The figure shows three views and two pictorial views of one solid part (mm, origin at its lowest corner). Answer the questions. A direction names the side the tool comes from. Give positions to 0.01 mm unless a question says otherwise; leave off trailing zeros. Loops run counter-clockwise (first coordinate to the right, second up) from the corner with the lowest first, then second, coordinate; pieces in that order, holes last. Notation, with made-up numbers: (75.5, -28.75) -> (113.5, -28.75) arc R21 cw to (113.5, -24.75) -> close; hole circle Ø9 at (72, 39.25). An arc over 180 degrees is marked (long way). Answer as CSV lines item,"result". Start each with the question number.
1. Flat-ended cylindrical pins translate along their axes: pin 1 Ø2.5 at (x, z) = (10, 10) entering from +Y; pin 2 Ø6 at (x, y) = (14.5, 2.5) entering from +Z; pin 3 Ø6 at (x, y) = (10.5, 1.5) entering from -Z; pin 4 Ø2 at (x, z) = (16.5, 3) entering from -Y. Find the tip coordinate at first contact, or state that the pin passes through.
2. Determine the mould class of the marked faces 3, 4, 5 and 6 for opening direction X: +X half, -X half, draft (parallel to the pull), parting line (faces both ways), or undercut.
3. Find section A-A, the plane z = 10. Give the vertices of the cut face in (x, y).
4. Find section D-D, the plane z = 12. Give the vertices of the cut face in (x, y).
5. A tool of negligible diameter and unlimited length cuts with its end or side. For the marked faces 1 and 2, from which of +Z, -Z, +X, -X, +Y, -Y can it reach the whole face along a straight path? Write none if from no direction.
6. Find the intervals of material crossed by line 1 along Y through (x, z) = (12, 4.5); line 2 along X through (y, z) = (2.25, 8.75) (1 decimal); line 3 along X through (y, z) = (9.25, 13), in increasing order.
7. Find section C-C, the plane y = 2. Give the vertices of the cut face in (x, z) (1 decimal).
8. Find section B-B, the plane x = 10. Give the vertices of the cut face in (y, z).
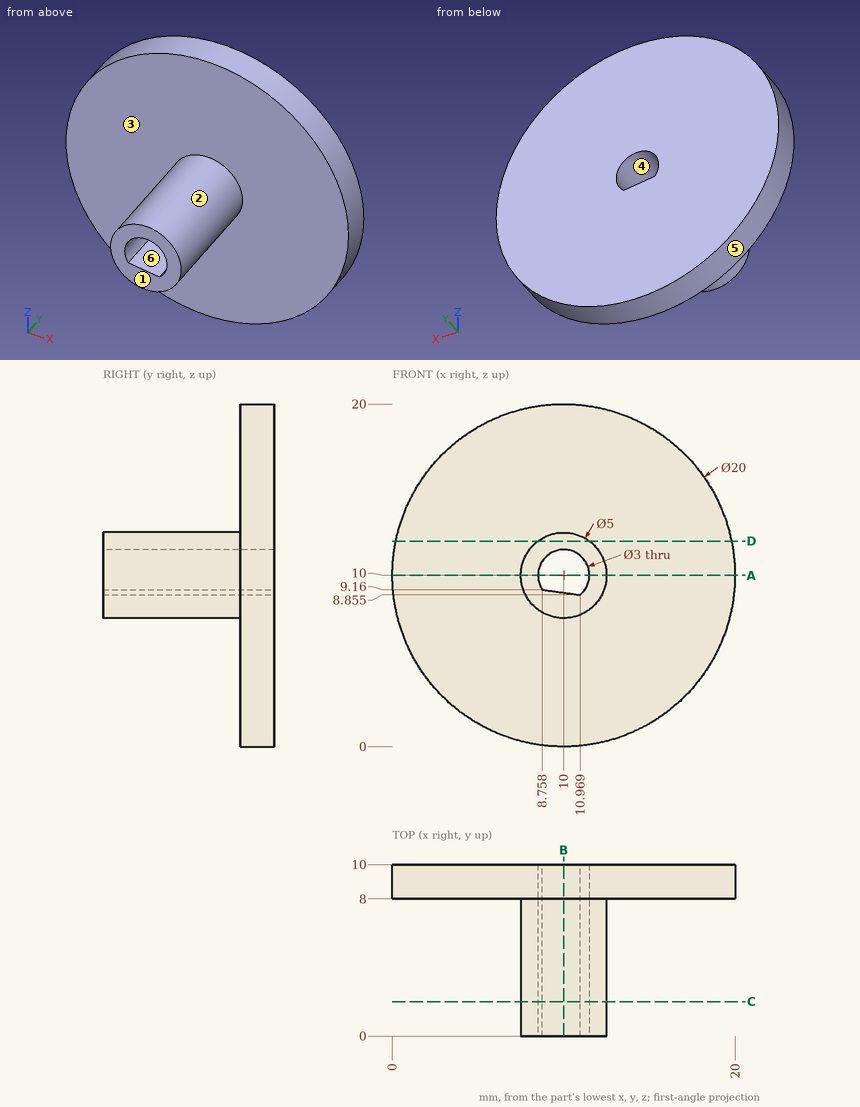
Resolved:
1,pin 1,"stops at y = 10"
1,pin 2,"stops at z = 12"
1,pin 3,"stops at z = 7.5"
1,pin 4,"stops at y = 8"
2,face 3,"draft"
2,face 4,"undercut"
2,face 5,"parting line"
2,face 6,"undercut"
3,outline,"(0, 8) -> (7.5, 8) -> (7.5, 0) -> (8.5, 0) -> (8.5, 10) -> (0, 10) -> close; (11.5, 0) -> (12.5, 0) -> (12.5, 8) -> (20, 8) -> (20, 10) -> (11.5, 10) -> close"
4,outline,"(0.2, 8) -> (8.5, 8) -> (8.5, 0) -> (11.5, 0) -> (11.5, 8) -> (19.8, 8) -> (19.8, 10) -> (0.2, 10) -> close"
5,face 1,"+Z, -Z, +X, -X, -Y"
5,face 2,"-Y"
6,line 1,"y = 8 to 10"
6,line 2,"x = 7.8 to 12.2"
6,line 3,"x = 0.46 to 19.54"
7,outline,"circle Ø5 at (10, 10); hole (8.8, 9.2) -> (11, 8.9) arc R1.5 ccw (long way) to start"
8,outline,"(0, 7.5) -> (8, 7.5) -> (8, 0) -> (10, 0) -> (10, 8.99) -> (0, 8.99) -> close; (0, 11.5) -> (10, 11.5) -> (10, 20) -> (8, 20) -> (8, 12.5) -> (0, 12.5) -> close"
